Design review of the part built by this model. Coordinates are the model's own, in mm. A direction names the side the tool comes from. Round coordinates to 2 decimals unless told otherwise and drop trailing zeros. Order: outer loops, then holes, each group sorted by start corner. A loop starts at its lowest first (then second) coordinate and runs counter-clockwise, first axis right, second up. Notation, with made-up numbers: (19, -11) - (34, -11) arc R28 cw to (34, 27) - close; hole circle Ø4 at (-34, -5). An arc over 180 degrees is marked (long way). Write item = value, one per line.
from build123d import *

# Parameters (mm, degrees)
F0_W     = 135.262012
F0_H     = 95.015392
F1_DEPTH = 25.4
F2_R     = 38.939289
F3_DEPTH = 31.75
F4_R     = 31.180051
F5_DEPTH = 76.2


with BuildPart() as f1:
    # F0 (on Front) → F1 (new body)
    with BuildSketch(Plane.XZ):
        Rectangle(F0_W, F0_H)
    extrude(amount=F1_DEPTH)

    # F2 (on face) → F3 (join)
    with BuildSketch(Plane.XZ.offset(25.4)):
        Circle(F2_R)
    extrude(amount=F3_DEPTH)

    # F4 (on Front) → F5 (cut)
    with BuildSketch(Plane.XZ):
        Circle(F4_R)
    extrude(amount=F5_DEPTH, mode=Mode.SUBTRACT)


solid = f1.part
1) We need section C-C on y = -10.5. Write out the cut boundary in (x, z), and give its area (3 significant figures).
Findings:
outline = (-67.63, -47.51) - (67.63, -47.51) - (67.63, 47.51) - (-67.63, 47.51) - close; hole circle Ø62.36 at (0, 0)
area = 9,800 mm^2
2) Clearance check with flat-ended pins moving along their axes: pin 1 Ø12 at (x, y) = (29, -37) entering from +Z; pin 2 Ø4 at (x, y) = (-19, -40.5) entering from +Z; pin 3 Ø6 at (y, z) = (-40.5, 1) entering from -X. State where each tip first meets the part, or that it passes through.
Findings:
pin_1 = 31.42
pin_2 = 35.03
pin_3 = -38.94
3) We need section B-B on z = 0. Write out the cut boundary in (x, y), and give its area (3 significant figures).
Findings:
outline = (-67.63, -25.4) - (-38.94, -25.4) - (-38.94, -57.15) - (-31.18, -57.15) - (-31.18, 0) - (-67.63, 0) - close; (31.18, -57.15) - (38.94, -57.15) - (38.94, -25.4) - (67.63, -25.4) - (67.63, 0) - (31.18, 0) - close
area = 2,340 mm^2
4) The part is to be moulded in two halves that separate along Z. For faces 1 (the flat face through (-1, -13, -47.508)), 2 (the cylindrical face through (-4.059, -28.175, 30.915)), 3 (the flat face through (-29, -57.15, 12)), 4 (the flat face through (-1, -13, 47.508)), say which applies: released by +Z, released by -Z, zero draft, split by the parting line, or undercut.
Findings:
face_1 = released by -Z
face_2 = undercut
face_3 = zero draft
face_4 = released by +Z
5) We need section D-D on z = 36.5. Write out the cut boundary in (x, y), and give its area (3 significant figures).
Findings:
outline = (-67.63, -25.4) - (-13.57, -25.4) - (-13.57, -57.15) - (13.57, -57.15) - (13.57, -25.4) - (67.63, -25.4) - (67.63, 0) - (-67.63, 0) - close
area = 4,300 mm^2
6) To check wall thickness, follow L1, parallel to X at y = -24, z = 0; L2, parallel to Z at x = 0, y = -28; L3, parallel to Y at x = 31, z = 29. State the ranges of each line that lie inside material, in increasing order. Write a range as from..to.
Findings:
L1 = -67.63..-31.18, 31.18..67.63
L2 = -38.94..-31.18, 31.18..38.94
L3 = -25.4..0
7) For faces 5 (the flat face through (-1, -25.4, -42)), 6 (the flat face through (-1, 0, 32)), list the 3-axis set-ups (+Z, -Z, +X, -X, +Y, -Y) from which the entire face can be reached by the end or side of a thin tool; tool diameter is ignored.
Findings:
face_5 = -Y
face_6 = +Z, -Z, +X, -X, +Y
8) We need section A-A on x = 0. Write out the cut boundary in (y, z), and give its area (3 significant figures).
Findings:
outline = (-57.15, -38.94) - (-25.4, -38.94) - (-25.4, -47.51) - (0, -47.51) - (0, -31.18) - (-57.15, -31.18) - close; (-57.15, 31.18) - (0, 31.18) - (0, 47.51) - (-25.4, 47.51) - (-25.4, 38.94) - (-57.15, 38.94) - close
area = 1,320 mm^2
